from build123d import *

# Parameters (mm, degrees)
SKETCH_1_W       = 90
SKETCH_1_H       = 88
TRAY_DEPTH       = 40
TRAYCAVITY_START = 3
SKETCH_2_W       = 86
SKETCH_2_H       = 84
TRAYCAVITY_DEPTH = 37


with BuildPart() as part:
    # 草图1 → Tray (new body)
    with BuildSketch(Plane.XY):
        with Locations((165, 0)):
            Rectangle(SKETCH_1_W, SKETCH_1_H)
    extrude(amount=TRAY_DEPTH)

    # 草图2 → TrayCavity (cut)
    with BuildSketch(Plane.XY.offset(TRAYCAVITY_START)):
        with Locations((165, 0)):
            Rectangle(SKETCH_2_W, SKETCH_2_H)
    extrude(amount=TRAYCAVITY_DEPTH, mode=Mode.SUBTRACT)


solid = part.part
Verification items for the finished model (mm, model axes). A direction names the side the tool comes from. Coordinates: 2 decimals unless noted, no trailing zeros. Write each loop counter-clockwise with the first axis right and the second up, starting at its lowest first coordinate (ties: lowest second). Pieces come first, ordered by that corner, then holes. Notation, with made-up numbers: (-17.75, 52) -> (18.25, 52) arc R15 ccw to (18.25, 71) -> close; hole circle Ø3 at (7.25, -36). An arc over 180 degrees is marked (long way). One line per item, written item: value. Start each with the question number.
Q1. Cross-section at C-C on x = 191. Enter the section's corners in (y, z).
Q2. Access from +Z, -Z, +X, -X, +Y, -Y to the whole of each face (thin tool, end or side, straight path). Record for faces 4 (the flat face through (120, -1, 20)), 5 (the flat face through (122, -1, 21)).
Q3. Mould release check, pull along X, two halves, no side actions. Record for faces 1 (the flat face through (161.5, -42.2, 40)), 2 (the flat face through (208, -1, 21)), 3 (the flat face through (210, -1, 20)): pulls with the +X half, pulls with the -X half, needs draft (parallel to the pull), parting line crosses it, or undercut.
Q4. Cross-section at A-A on z = 18. Enter the section's corners in (x, y).
Q5. Cross-section at B-B on y = -25.5. Enter the section's corners in (x, z), and give its area (3 significant figures).
Q6. Go/stop test with a flat-tipped pin: P1, Ø5, axis at x = 131, y = -12.5, coming from the +Z side. Record where the tip stops, or that it passes through.
Q7. Thickness scan on L1, parallel to Y at x = 205.5, z = 17; L2, parallel to X at y = 27.5, z = 16.5; L3, parallel to Z at x = 129, y = -7.5. Record the ranges inside material, lowest first. Write a range as from..to.
Checked values:
1. outline: (-44, 0) -> (44, 0) -> (44, 40) -> (42, 40) -> (42, 3) -> (-42, 3) -> (-42, 40) -> (-44, 40) -> close
2. face 4: +Z, -Z, -X, +Y, -Y
2. face 5: +Z
3. face 1: needs draft
3. face 2: undercut
3. face 3: pulls with the +X half
4. outline: (120, -44) -> (210, -44) -> (210, 44) -> (120, 44) -> close; hole (122, -42) -> (208, -42) -> (208, 42) -> (122, 42) -> close
5. outline: (120, 0) -> (210, 0) -> (210, 40) -> (208, 40) -> (208, 3) -> (122, 3) -> (122, 40) -> (120, 40) -> close
5. area: 418 mm²
6. P1: stops at z = 3
7. L1: y = -44..-42, 42..44
7. L2: x = 120..122, 208..210
7. L3: z = 0..3
